Could you check a few things on this model? Use its own coordinates, in mm. Coordinates: 2 decimals unless noted, no trailing zeros. Order: outer loops, then holes, each group sorted by start corner. A loop starts at its lowest first (then second) coordinate and runs counter-clockwise, first axis right, second up. Notation, with made-up numbers: (88.5, 51.25) -> (111.5, 51.25) arc R18 cw to (111.5, 61.25) -> close; hole circle Ø10 at (-30.75, 41.25). An arc over 180 degrees is marked (long way). Use a Markdown table: item, result. Add a question column.
1) Will these pins go through, and if not, where does the flat tip stop? pin 1 Ø7 at (x, z) = (3, 1193) entering from -Y; pin 2 Ø12 at (y, z) = (4.5, 1477) entering from -X; pin 3 Ø9 at (y, z) = (1.5, 1563) entering from +X; pin 4 Ø1.5 at (x, y) = (3.5, 5.5) entering from -Z.
2) If we section it at A-A (x = -3.5): Write out the boundary of the cut face in (y, z), plus the area to 3 significant figures.
3) If we section it at B-B (z = 405.5): Write out the boundary of the cut face in (x, y), plus the area to 3 significant figures.
4) If I drill on L1, parallel to Y at x = 11.5, z = 1362; L2, parallel to Z at x = -8, y = 6.5, over which ranges is the centre line in solid material (lowest first)? Write a range as [from, to].
```python
from build123d import *

# Parameters (mm, degrees)
SCHIZZO1_W                   = 50
SCHIZZO1_H                   = 50
ESTRUSIONE_ESTRUSIONE1_DEPTH = 5
SCHIZZO2_W                   = 30
SCHIZZO2_H                   = 30
SCHIZZO2_W_2                 = 24
SCHIZZO2_H_2                 = 24
ESTRUSIONE_ESTRUSIONE2_DEPTH = 2205
SCHIZZO3_W                   = 24
SCHIZZO3_H                   = 24
ESTRUSIONE_ESTRUSIONE3_DEPTH = 5


with BuildPart() as part:
    # Schizzo1 → Estrusione-Estrusione1 (new body)
    with BuildSketch(Plane.XY):
        Rectangle(SCHIZZO1_W, SCHIZZO1_H)
    extrude(amount=ESTRUSIONE_ESTRUSIONE1_DEPTH)

    # Schizzo2 → Estrusione-Estrusione2 (add)
    with BuildSketch(Plane.XY.offset(5)):
        Rectangle(SCHIZZO2_W, SCHIZZO2_H)
        Rectangle(SCHIZZO2_W_2, SCHIZZO2_H_2, mode=Mode.SUBTRACT)
    extrude(amount=ESTRUSIONE_ESTRUSIONE2_DEPTH)

    # Schizzo3 → Estrusione-Estrusione3 (add)
    with BuildSketch(Plane.XY.offset(2210)):
        Rectangle(SCHIZZO3_W, SCHIZZO3_H)
    extrude(amount=-ESTRUSIONE_ESTRUSIONE3_DEPTH)


solid = part.part
```
Answer sheet:
| question | item | result |
|---|---|---|
| 1 | pin 1 | y = -15 |
| 1 | pin 2 | x = -15 |
| 1 | pin 3 | x = 15 |
| 1 | pin 4 | z = 0 |
| 2 | outline | (-25, 0) -> (25, 0) -> (25, 5) -> (15, 5) -> (15, 2210) -> (-15, 2210) -> (-15, 5) -> (-25, 5) -> close; hole (-12, 5) -> (12, 5) -> (12, 2205) -> (-12, 2205) -> close |
| 2 | area | 13,600 mm2 |
| 3 | outline | (-15, -15) -> (15, -15) -> (15, 15) -> (-15, 15) -> close; hole (-12, -12) -> (12, -12) -> (12, 12) -> (-12, 12) -> close |
| 3 | area | 324 mm2 |
| 4 | L1 | [-15, -12], [12, 15] |
| 4 | L2 | [0, 5], [2205, 2210] |
